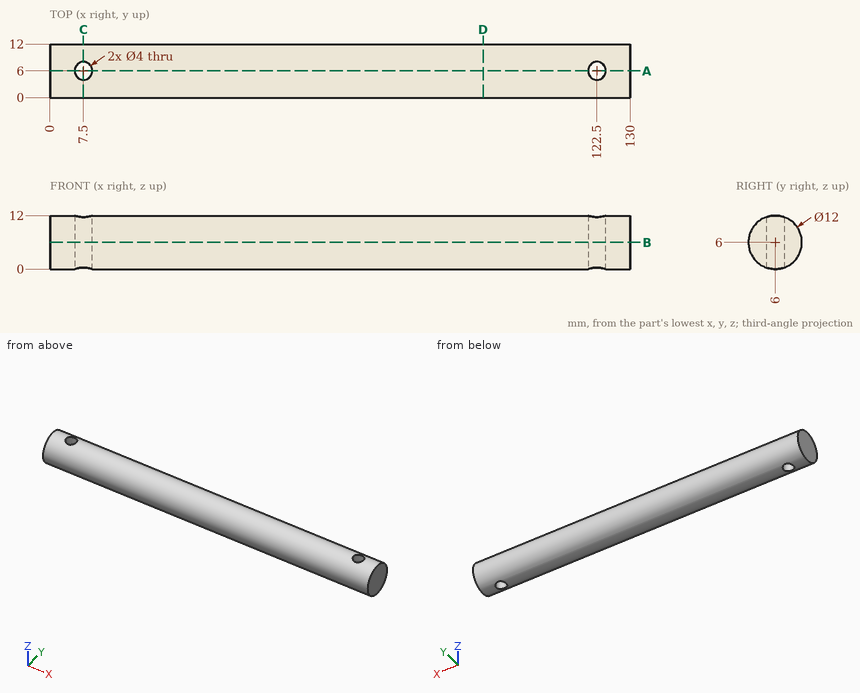
The drawing under review shows one solid part. Ordinate dimensions are in mm from its lowest x, y, z. Give positions to 0.01 mm unless a question says otherwise; leave off trailing zeros. Write each loop counter-clockwise with the first axis right and the second up, starting at its lowest first coordinate (ties: lowest second). Pieces come first, ordered by that corner, then holes.
1. Add section A-A, the plane y = 6. Write out the cut boundary in (x, z), plus the area to 3 significant figures.
2. Add section C-C, the plane x = 7.5. Write out the cut boundary in (y, z).
3. For P1, Ø2, axis at x = 40.5, y = 8.5, coming from the +Z side; P2, Ø1.5, axis at x = 44.5, z = 7, coming from the -Y side; P3, Ø6, axis at x = 103.5, y = 2.5, coming from the +Z side, all flat-tipped, find the tip position at first contact; note any pin that passes through.
4. Wall thickness on L1, parallel to X at y = 6.25, z = 9.5; L2, parallel to Y at x = 7.5, z = 6; L3, parallel to Y at x = 122.5, z = 8: over which ranges is each line inside the solid? List them lowest first.
5. Add section D-D, the plane x = 97. Write out the cut boundary in (y, z).
6. Add section B-B, the plane z = 6. Write out the cut boundary in (x, y), plus the area to 3 significant figures.
Worked answers:
1. outline: (0, 0) - (5.5, 0) - (5.5, 12) - (0, 12) - close; (9.5, 0) - (120.5, 0) - (120.5, 12) - (9.5, 12) - close; (124.5, 0) - (130, 0) - (130, 12) - (124.5, 12) - close
1. area: 1,460 mm2
2. outline: (4, 0.34) - (4, 11.66) arc R6 ccw to start; (8, 0.34) arc R6 ccw to (8, 11.66) - close
3. P1: stops at z = 11.81
3. P2: stops at y = 0.01
3. P3: stops at z = 11.98
4. L1: x = 0 to 5.52, 9.48 to 120.52, 124.48 to 130
4. L2: y = 0 to 4, 8 to 12
4. L3: y = 0.34 to 4, 8 to 11.66
5. outline: circle Ø12 at (6, 6)
6. outline: (0, 0) - (130, 0) - (130, 12) - (0, 12) - close; hole circle Ø4 at (7.5, 6); hole circle Ø4 at (122.5, 6)
6. area: 1,530 mm2
